```python
from build123d import *

# Parameters (mm, degrees)
BOSS_EXTRUDE1_DEPTH = 1.5875
CUT_EXTRUDE3_DEPTH  = 10


with BuildPart() as part:
    # Sketch1 → Boss-Extrude1 (new, symmetric)
    with BuildSketch(Plane.XY):
        Polygon((0, 0), (5, 0), (5, -3.175), (11, -3.175), (11, 0), (19, 0), (19, 9), (9, 9), (9, 19), (0, 19), (0, 11), (-3.175, 11), (-3.175, 5), (0, 5), align=None)
    extrude(amount=BOSS_EXTRUDE1_DEPTH, both=True)

    # Sketch2 → Cut-Extrude3 (cut, symmetric)
    with BuildSketch(Plane(origin=(0, 9, 0), x_dir=(1, 0, 0), z_dir=(0, 1, 0))):
        Polygon((21.145490005, 0), (19, 0), (19, -1.5875), (17.4125, -1.5875), (19.19836718, -4.188524989), align=None)
        Polygon((19, 1.5875), (19, 0), (21.145490005, 0), (20.434145586, 3.927655586), (17.4125, 1.5875), align=None)
        Polygon((19, -1.5875), (19, 0), (17.4125, -1.5875), align=None)
        Polygon((17.4125, 1.5875), (19, 0), (19, 1.5875), align=None)
    extrude(amount=CUT_EXTRUDE3_DEPTH, both=True, mode=Mode.SUBTRACT)


solid = part.part
```
Design review of the part built by this model. Coordinates are the model's own, in mm. A direction names the side the tool comes from. Give positions to 0.01 mm unless a question says otherwise; leave off trailing zeros. Order: outer loops, then holes, each group sorted by start corner. A loop starts at its lowest first (then second) coordinate and runs counter-clockwise, first axis right, second up. Notation, with made-up numbers: (32.25, 64.5) -> (55.25, 64.5) arc R13 ccw to (55.25, 85.5) -> close; hole circle Ø4 at (-34.75, -11). An arc over 180 degrees is marked (long way). Write item = value, one per line. Start each with the question number.
(1) We need section C-C on x = 10.25. Write out the cut boundary in (y, z) (1 decimal).
(2) We need section D-D on z = -1. Write out the cut boundary in (x, y) (3 decimals), plus the area to 3 significant figures.
(3) To check wall thickness, follow line 1 along Y through (x, z) = (11.75, -0.4); line 2 along Y through (x, z) = (4.75, 0.65). State the ranges of each line that lie inside material, in increasing order.
(4) We need section A-A on z = 0.95. Write out the cut boundary in (x, y) (3 decimals), plus the area to 3 significant figures.
(5) We need section B-B on y = 6.5. Write out the cut boundary in (x, z) (1 decimal), plus the area to 3 significant figures.
(6) For faces 1 (the face through (11, -2, 0)), 2 (the face through (5, -2, 0)), 3 (the face through (0, 15, 0)), 4 (the face through (9, 14, 0)), list the 3-axis set-ups (+Z, -Z, +X, -X, +Y, -Y) from which the entire face can be reached by the end or side of a thin tool; tool diameter is ignored.
(7) For pin 1 (1 mm diameter, centred on y = 12, z = 1, fed in from +X); pin 2 (1.6 mm diameter, centred on x = 1.5, z = -0.5, fed in from -Y); pin 3 (1.6 mm diameter, centred on y = -2, z = 0, fed in from -X), all flat-tipped, find the tip position at first contact; note any pin that passes through.
Numbers:
q1.outline = (-3.2, -1.6) -> (9, -1.6) -> (9, 1.6) -> (-3.2, 1.6) -> close
q2.outline = (-3.175, 5) -> (0, 5) -> (0, 0) -> (5, 0) -> (5, -3.175) -> (11, -3.175) -> (11, 0) -> (18, 0) -> (18, 9) -> (9, 9) -> (9, 19) -> (0, 19) -> (0, 11) -> (-3.175, 11) -> close
q2.area = 290 mm^2
q3.line_1 = 0 to 9
q3.line_2 = 0 to 19
q4.outline = (-3.175, 5) -> (0, 5) -> (0, 0) -> (5, 0) -> (5, -3.175) -> (11, -3.175) -> (11, 0) -> (18.05, 0) -> (18.05, 9) -> (9, 9) -> (9, 19) -> (0, 19) -> (0, 11) -> (-3.175, 11) -> close
q4.area = 291 mm^2
q5.outline = (-3.2, -1.6) -> (17.4, -1.6) -> (19, 0) -> (17.4, 1.6) -> (-3.2, 1.6) -> close
q5.area = 67.9 mm^2
q6.face_1 = +Z, -Z, +X, -Y
q6.face_2 = +Z, -Z, -X, -Y
q6.face_3 = +Z, -Z, -X, +Y
q6.face_4 = +Z, -Z, +X, +Y
q7.pin_1 = 9
q7.pin_2 = 0
q7.pin_3 = 5
